Work out the finished part from the listing and answer in its coordinate system (mm). A direction names the side the tool comes from. Give positions to 0.01 mm unless a question says otherwise; leave off trailing zeros. Loops run counter-clockwise (first coordinate to the right, second up) from the corner with the lowest first, then second, coordinate; pieces in that order, holes last. Notation, with made-up numbers: M -25.75,52 L 11.25,52 A25 cw 11.25,88 Z; hole C -33,73 d8. An arc over 180 degrees is marked long. Answer as a JSON object with one key per item and string values. Group by question number.
```python
from build123d import *

# Parameters (mm, degrees)
ESQUISSE1_W                   = 30.8
ESQUISSE1_H                   = 24.15
BOSS_EXTRU_1_DEPTH            = 22
ENL_V_START                   = -22
ENL_V_MAT_EXTRU_2_DEPTH       = 22
ESQUISSE3_R                   = 1.5
ENL_V_MAT_EXTRU_3_DEPTH       = 4.4
ESQUISSE6_R                   = 3.2
ENL_V_MAT_EXTRU_6_DEPTH       = 3.4
ESQUISSE7_R                   = 3.2
ENL_V_MAT_EXTRU_7_DEPTH       = 3.4
ESQUISSE10_R                  = 3.2
ENL_V_MAT_EXTRU_10_DEPTH      = 3.4
ESQUISSE11_R                  = 3.2
ENL_V_MAT_EXTRU_11_DEPTH      = 3.4
ENL_V_MAT_EXTRU_14_DEPTH      = 47.950397903
ENL_V_MAT_EXTRU_14_DEPTH_BACK = 4.8
ENL_V_MAT_EXTRU_19_DEPTH      = 4.8
ENL_V_MAT_EXTRU_20_DEPTH      = 4.8
ENL_V_MAT_EXTRU_21_DEPTH      = 4.8


# Read off the part's stored shape, not the designer's step: Enlèv. mat.-Extru.2
with BuildPart() as part:
    # Esquisse1 → Boss.-Extru.1 (new body)
    with BuildSketch(Plane.XY):
        with Locations((-20.769736842, 6.111184211)):
            Rectangle(ESQUISSE1_W, ESQUISSE1_H)
    extrude(amount=BOSS_EXTRU_1_DEPTH)

    # Enlèv. mat.-Extru.2 outline → Enlèv. mat.-Extru.2 (cut)
    with BuildSketch(Plane.XY.offset(22).offset(ENL_V_START)):
        Polygon((-30.869736842, -5.963815789), (-10.669736842, -5.963815789), (-10.669736842, -2.113815789), (-16.919736842, -2.113815789), (-16.919736842, 2.686184211), (-10.669736842, 2.686184211), (-10.669736842, 10.386184211), (-18.369736842, 10.386184211), (-18.369736842, 4.136184211), (-23.169736842, 4.136184211), (-23.169736842, 10.386184211), (-30.869736842, 10.386184211), (-30.869736842, 2.686184211), (-24.619736842, 2.686184211), (-24.619736842, -2.113815789), (-30.869736842, -2.113815789), align=None)
    extrude(amount=ENL_V_MAT_EXTRU_2_DEPTH, mode=Mode.SUBTRACT)

    # Esquisse3 → Enlèv. mat.-Extru.3 (cut)
    with BuildSketch(Plane(origin=(0, 18.186184211, 0), x_dir=(1, 0, 0), z_dir=(0, 1, 0))):
        with Locations(Location((-26.424736842, -5.345, 0), (0, 0, 270))):
            Circle(ESQUISSE3_R)
        with Locations(Location((-15.114736842, -5.345, 0), (0, 0, 270))):
            Circle(ESQUISSE3_R)
        with Locations(Location((-26.424736842, -16.655, 0), (0, 0, 270))):
            Circle(ESQUISSE3_R)
        with Locations(Location((-15.114736842, -16.655, 0), (0, 0, 270))):
            Circle(ESQUISSE3_R)
    extrude(amount=-ENL_V_MAT_EXTRU_3_DEPTH, mode=Mode.SUBTRACT)

    # Esquisse6 → Enlèv. mat.-Extru.6 (cut)
    with BuildSketch(Plane(origin=(0, 13.786184211, 0), x_dir=(1, 0, 0), z_dir=(0, 1, 0))):
        with Locations(Location((-15.126255276, -16.627264665, 0), (0, 0, 270))):
            Circle(ESQUISSE6_R)
    extrude(amount=-ENL_V_MAT_EXTRU_6_DEPTH, mode=Mode.SUBTRACT)

    # Esquisse7 → Enlèv. mat.-Extru.7 (cut)
    with BuildSketch(Plane(origin=(0, 13.786184211, 0), x_dir=(1, 0, 0), z_dir=(0, 1, 0))):
        with Locations(Location((-26.44565221, -16.692132269, 0), (0, 0, 270))):
            Circle(ESQUISSE7_R)
    extrude(amount=-ENL_V_MAT_EXTRU_7_DEPTH, mode=Mode.SUBTRACT)

    # Esquisse10 → Enlèv. mat.-Extru.10 (cut)
    with BuildSketch(Plane(origin=(0, 13.786184211, 0), x_dir=(1, 0, 0), z_dir=(0, 1, 0))):
        with Locations(Location((-15.114736842, -5.345, 0), (0, 0, 270))):
            Circle(ESQUISSE10_R)
    extrude(amount=-ENL_V_MAT_EXTRU_10_DEPTH, mode=Mode.SUBTRACT)

    # Esquisse11 → Enlèv. mat.-Extru.11 (cut)
    with BuildSketch(Plane(origin=(0, 13.786184211, 0), x_dir=(1, 0, 0), z_dir=(0, 1, 0))):
        with Locations(Location((-26.424736842, -5.345, 0), (0, 0, 270))):
            Circle(ESQUISSE11_R)
    extrude(amount=-ENL_V_MAT_EXTRU_11_DEPTH, mode=Mode.SUBTRACT)

    # Esquisse12 → Enlèv. mat.-Extru.14 (cut, two sides: drawn at the far end of the back side and taken through both)
    with BuildSketch(Plane(origin=(0, -2.113815789, 0), x_dir=(-1, 0, 0), z_dir=(0, -1, 0)).offset(-ENL_V_MAT_EXTRU_14_DEPTH_BACK)):
        Polygon((16.919736842, -9), (16.919736842, -2), (13.419736842, -2), (10.669736842, -3.636306817), (10.669736842, -7.363693183), (13.419736842, -9), align=None)
    extrude(amount=ENL_V_MAT_EXTRU_14_DEPTH + ENL_V_MAT_EXTRU_14_DEPTH_BACK, mode=Mode.SUBTRACT)

    # Esquisse13 → Enlèv. mat.-Extru.19 (cut)
    with BuildSketch(Plane(origin=(0, -2.113815789, 0), x_dir=(-1, 0, 0), z_dir=(0, -1, 0))):
        Polygon((24.619736842, -2), (28.119736842, -2), (30.869736842, -3.636306817), (30.869736842, -7.363693183), (28.119736842, -9), (24.619736842, -9), align=None)
    extrude(amount=-ENL_V_MAT_EXTRU_19_DEPTH, mode=Mode.SUBTRACT)

    # Esquisse14 → Enlèv. mat.-Extru.20 (cut)
    with BuildSketch(Plane(origin=(0, -2.113815789, 0), x_dir=(-1, 0, 0), z_dir=(0, -1, 0))):
        Polygon((24.619736842, -20), (28.119736842, -20), (30.869736842, -18.363693183), (30.869736842, -14.636306817), (28.119736842, -13), (24.619736842, -13), align=None)
    extrude(amount=-ENL_V_MAT_EXTRU_20_DEPTH, mode=Mode.SUBTRACT)

    # Esquisse16 → Enlèv. mat.-Extru.21 (cut)
    with BuildSketch(Plane(origin=(0, -2.113815789, 0), x_dir=(-1, 0, 0), z_dir=(0, -1, 0))):
        Polygon((16.919736842, -20), (13.419736842, -20), (10.669736842, -18.363693183), (10.669736842, -14.636306817), (13.419736842, -13), (16.919736842, -13), align=None)
    extrude(amount=-ENL_V_MAT_EXTRU_21_DEPTH, mode=Mode.SUBTRACT)


solid = part.part
```
Item 1: A cutting plane is placed at D-D (z = 17.25). Determine the outline of the cut face in (x, y).
Item 2: A cutting plane is placed at A-A (y = 5.5). Determine the outline of the cut face in (x, z), and give its area (3 significant figures).
Item 3: For a pull along Z with two mould halves and no side action, classify faces 4 (the flat face through (-12.06, 0.32, 2.81)), 5 (the flat face through (-36.17, 6, 11)), 6 (the flat face through (-21, 9, 0)) as pulls with the +Z half, pulls with the -Z half, needs draft (parallel to the pull), parting line crosses it, or undercut.
Item 4: Find the intervals of material crossed by probe 1 along X at (y, z) = (8.25, 1.75); probe 2 along Z at (x, y) = (-27, -1); probe 3 along X at (y, z) = (3.25, 18), in increasing order. Write a range as [from, to].
Item 5: Given pin 1 Ø1.4 at (x, z) = (-21.5, 10) entering from -Y; pin 2 Ø3 at (x, z) = (-16, 6) entering from -Y; pin 3 Ø4 at (x, z) = (-27.5, 1) entering from -Y, each flat-ended and moving along its own axis, determine where each tip first touches the part or whether it passes through.
Item 6: A tool of negligible diameter and unlimited length cuts with its end or side. For faces 1 (the flat face through (-14, 2.686, 1)), 2 (the flat face through (-10.67, 4, 11)), 3 (the flat face through (-12.06, 0.25, 19.19)), from which of +Z, -Z, +X, -X, +Y, -Y can it reach the whole face along a straight path? Write none if from no direction.
Item 7: A cutting plane is placed at C-C (x = -28.5). Determine the outline of the cut face in (y, z), and give its area (3 significant figures).
The answers:
{
 "1": {"outline": "M -36.17,-5.96 L -30.87,-5.96 L -30.87,10.39 L -29.6,10.39 L -29.6,13.79 L -27.8,13.79 L -27.8,18.19 L -36.17,18.19 Z; M -25.05,13.79 L -23.29,13.79 L -23.29,10.39 L -23.17,10.39 L -23.17,4.14 L -18.37,4.14 L -18.37,10.39 L -18.27,10.39 L -18.27,13.79 L -16.49,13.79 L -16.49,18.19 L -25.05,18.19 Z; M -13.74,13.79 L -11.99,13.79 L -11.99,10.39 L -10.67,10.39 L -10.67,-5.96 L -5.37,-5.96 L -5.37,18.19 L -13.74,18.19 Z"},
 "2": {"outline": "M -36.17,0 L -30.87,0 L -30.87,22 L -36.17,22 Z; M -23.17,0 L -18.37,0 L -18.37,22 L -23.17,22 Z; M -10.67,0 L -5.37,0 L -5.37,22 L -10.67,22 Z", "area": "339 mm^2"},
 "3": {"face 4": "undercut", "face 5": "needs draft", "face 6": "pulls with the -Z half"},
 "4": {"probe 1": "x = [-36.17, -30.87], [-23.17, -18.37], [-10.67, -5.37]", "probe 2": "z = [0, 2], [9, 13], [20, 22]", "probe 3": "x = [-36.17, -30.87], [-10.67, -5.37]"},
 "5": {"pin 1": "stops at y = 4.14", "pin 2": "stops at y = 13.79", "pin 3": "stops at y = -2.11"},
 "6": {"face 1": "+Z, -Z", "face 2": "none", "face 3": "-Y"},
 "7": {"outline": "M -2.11,0 L 2.69,0 L 2.69,2.23 L -2.11,2.23 Z; M -2.11,8.77 L 2.69,8.77 L 2.69,13.23 L -2.11,13.23 Z; M -2.11,19.77 L 2.69,19.77 L 2.69,22 L -2.11,22 Z; M 10.39,0 L 18.19,0 L 18.19,22 L 10.39,22 L 10.39,19.15 L 13.79,19.15 L 13.79,14.24 L 10.39,14.24 L 10.39,7.78 L 13.79,7.78 L 13.79,2.91 L 10.39,2.91 Z", "area": "181 mm^2"}
}
